Geometry check sheet. Reference: the model listing, model coordinates, mm. Face numbers are marked on the shaded views. A direction names the side the tool comes from. Coordinates: 2 decimals unless noted, no trailing zeros. Order: outer loops, then holes, each group sorted by start corner. A loop starts at its lowest first (then second) coordinate and runs counter-clockwise, first axis right, second up. Notation, with made-up numbers: (33.25, 76) - (70.25, 76) arc R14 cw to (70.25, 82) - close; hole circle Ø6 at (52, 1). An arc over 180 degrees is marked (long way). Return JSON: item names as keys, results as strings. Group by question number.
Item 1: Section check A-A on x = 0. Enter the section's corners in (y, z).
Item 2: Draft check along X on the marked faces 6, 7 and 8. Enter one of: pulls with the +X half, pulls with the -X half, needs draft (parallel to the pull), parting line crosses it, or undercut.
Item 3: Tool access check on the marked faces 1, 2, 3, 4 and 5. Record the directions out of +Z, -Z, +X, -X, +Y, -Y that give a thin tool (end or side, any length) a straight path to the whole face; none if there is none.
Item 4: Scan lines: probe 1 along X at (y, z) = (-1.5, 5.5); probe 2 along Y at (x, z) = (7.5, 2); probe 3 along X at (y, z) = (1.75, 0.75). Record each from-to range of solid material in increasing order.
Item 5: Section check B-B on z = 5. Give the number of separate pieces and of enclosed holes in the cut face, then the cut area to 3 significant figures.
Item 6: Gauge pin test, flat ends, axial feed: pin 1 (2 mm diameter, centred on x = 12, y = -0.5, fed in from -Z); pin 2 (4.5 mm diameter, centred on x = 12.5, z = 4.5, fed in from +Y); pin 3 (3 mm diameter, centred on x = 2.5, z = 7, fed in from +Y). Record the tip position at first contact, or that the pin passes through.
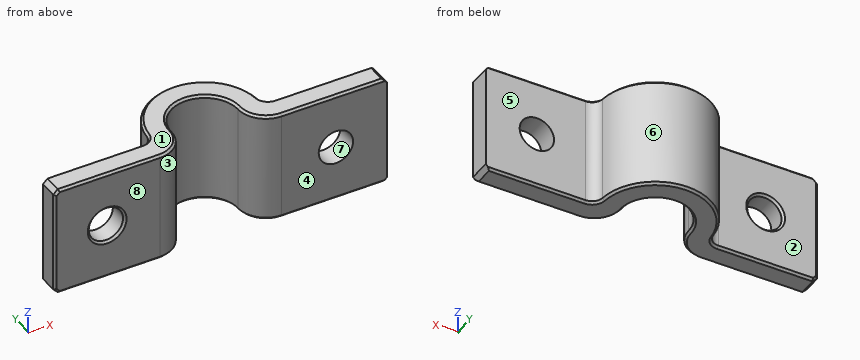
from build123d import *

# Parameters (mm, degrees)
EXTRUDE_3_DEPTH     = 10
FILLET_2_R          = 1
FILLET_3_R          = 2.5
CHAMFER_1_SIZE      = 0.4
SKETCH_5_R          = 1.55
CUT_EXTRUDE_2_DEPTH = 12
CHAMFER_2_SIZE      = 0.2


with BuildPart() as part:
    # 草图4 → 凸台-拉伸3 (new body)
    with BuildSketch(Plane.XY):
        with BuildLine():
            Line((-5, 0), (-5, -0.5))
            Line((-5, -0.5), (-15, -0.5))
            Line((-15, -0.5), (-15, -2.5))
            Line((-15, -2.5), (-5, -2.5))
            Line((-5, -2.5), (-3, -2.5))
            Line((-3, -2.5), (-3, 0))
            ThreePointArc((-3, 0), (0, 3), (3, 0))
            Line((3, 0), (3, -2.5))
            Line((3, -2.5), (5, -2.5))
            Line((5, -2.5), (15, -2.5))
            Line((15, -2.5), (15, -0.5))
            Line((15, -0.5), (5, -0.5))
            Line((5, -0.5), (5, 0))
            ThreePointArc((5, 0), (0, 5), (-5, 0))
        make_face()
    extrude(amount=EXTRUDE_3_DEPTH)

    # 圆角2
    fillet_2_edges = [part.edges().sort_by_distance(p)[0] for p in [
        (5, -0.5, 5),
        (-5, -0.5, 5),
    ]]
    fillet(fillet_2_edges, radius=FILLET_2_R)

    # 圆角3
    fillet_3_edges = [part.edges().sort_by_distance(p)[0] for p in [
        (-3, -2.5, 5),
        (3, -2.5, 5),
    ]]
    fillet(fillet_3_edges, radius=FILLET_3_R - 0.0001)  # a hair under: the kernel refuses the full size

    # 倒角1
    chamfer_1_edges = [part.edges().sort_by_distance(p)[0] for p in [
        (-15, -1.5, 0),
        (15, -1.5, 0),
        (15, -1.5, 10),
        (-15, -1.5, 10),
    ]]
    chamfer(chamfer_1_edges, length=CHAMFER_1_SIZE)

    # 草图5 → 切除-拉伸2 (cut)
    with BuildSketch(Plane(origin=(0, -0.5, 0), x_dir=(1, 0, 0), z_dir=(0, 1, 0))):
        with Locations(Location((-10.24814383, -5, 0), (0, 0, 180))):
            Circle(SKETCH_5_R)
        with Locations(Location((10.389565186, -5, 0), (0, 0, 180))):
            Circle(SKETCH_5_R)
    extrude(amount=-CUT_EXTRUDE_2_DEPTH, mode=Mode.SUBTRACT)

    # 倒角2
    chamfer_2_edges = [part.edges().sort_by_distance(p)[0] for p in [
        (0, 3, 0),
        (0, 5, 0),
        (0, 5, 10),
        (-10.289565186, -0.5, 0),
        (-10.289565186, -0.5, 10),
        (5.302127171, -0.235980072, 0),
        (5.302127171, -0.235980072, 10),
        (-5.302127171, -0.235980072, 0),
        (-5.302127171, -0.235980072, 10),
        (10.04995, -2.5, 0),
        (3.732203758, -1.767796242, 0),
        (-3.732203758, -1.767796242, 0),
        (10.04995, -2.5, 10),
        (3.732203758, -1.767796242, 10),
        (-3.732203758, -1.767796242, 10),
        (-10.04995, -2.5, 10),
        (10.289565186, -0.5, 10),
        (10.289565186, -0.5, 0),
        (-10.04995, -2.5, 0),
        (-15, -2.5, 5),
        (-14.8, -2.5, 0.2),
        (-14.8, -2.5, 9.8),
        (-15, -0.5, 5),
        (-14.8, -0.5, 0.2),
        (-14.8, -0.5, 9.8),
        (0, 3, 10),
        (-8.69814383, -2.5, 5),
        (-8.69814383, -0.5, 5),
    ]]
    chamfer(chamfer_2_edges, length=CHAMFER_2_SIZE)


solid = part.part
Computed:
{
 "1": {"outline": "(3, 0.2) - (3.2, 0) - (4.8, 0) - (5, 0.2) - (5, 9.8) - (4.8, 10) - (3.2, 10) - (3, 9.8) - close"},
 "2": {"face 6": "parting line crosses it", "face 7": "undercut", "face 8": "needs draft"},
 "3": {"face 1": "+Z, +X, -X, +Y, -Y", "face 2": "+Z, -Z, -X, +Y", "face 3": "+Z, -Z, -Y", "face 4": "+Z, -Z, +X, -X, -Y", "face 5": "+Z, -Z, +X, +Y"},
 "4": {"probe 1": "x = -15 to -11.72, -8.78 to -3.5, 3.5 to 8.92, 11.86 to 15", "probe 2": "y = -2.5 to -0.5", "probe 3": "x = -4.68 to -2.44, 2.44 to 4.68"},
 "5": {"separate pieces": "3", "enclosed holes": "0", "area": "60.3 mm²"},
 "6": {"pin 1": "stops at z = 0", "pin 2": "stops at y = -0.5", "pin 3": "stops at y = 4.9"}
}
